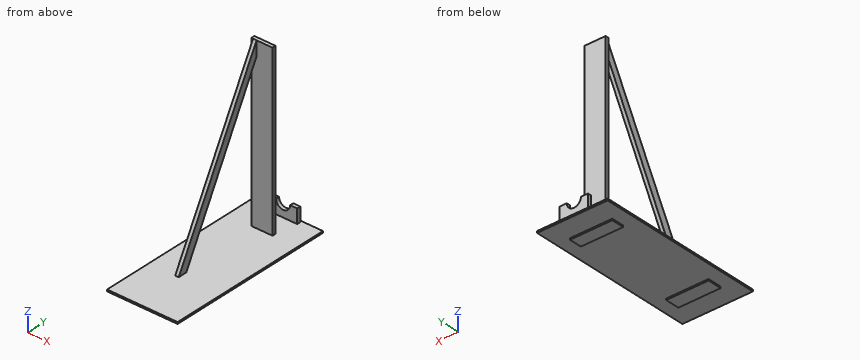
from build123d import *

# Parameters (mm, degrees)
F0_W      = 254
F0_H      = 609.6
F1_DEPTH  = 6.35
F2_W      = 152.4
F2_H      = 50.8
F2_H_2    = 45.6810940742
F3_DEPTH  = 5.08
F5_DEPTH  = 50.8
F6_W      = 76.2
F6_H      = 12.7
F7_DEPTH  = 609.6
F9_DEPTH  = 6.35
F11_DEPTH = 25.4


with BuildPart() as f1:
    # F0 (on Top) → F1 (new body)
    with BuildSketch(Plane.XY):
        with Locations((25.4, 0)):
            Rectangle(F0_W, F0_H)
    extrude(amount=F1_DEPTH)

    # F2 (on face) → F3 (join)
    with BuildSketch(Plane(origin=(0, 0, 0), x_dir=(1, 0, 0), z_dir=(0, 0, -1))):
        with Locations((25.4, 203.2)):
            Rectangle(F2_W, F2_H)
        with Locations((25.4, -203.2)):
            Rectangle(F2_W, F2_H_2)
    extrude(amount=F3_DEPTH)

    # F4 (on face) → F5 (join)
    with BuildSketch(Plane.XY.offset(6.35)):
        Polygon((76.2, 285.75), (76.2, 298.45), (25.4, 298.45), (-25.4, 298.45), (-25.4, 285.75), align=None)
    extrude(amount=F5_DEPTH)

    # F6 (on face) → F7 (join)
    with BuildSketch(Plane.XY.offset(6.35)):
        with Locations((25.4, 203.2)):
            Rectangle(F6_W, F6_H)
    extrude(amount=F7_DEPTH)

    # F8 (on Right) → F9 (join, symmetric)
    with BuildSketch(Plane.YZ):
        Polygon((-133.4145218134, 0), (-101.6, 0), (196.6719031334, 564.3243789673), (196.6719031334, 616.1219477654), align=None)
    extrude(amount=F9_DEPTH, both=True)

    # F10 (on face) → F11 (cut)
    with BuildSketch(Plane(origin=(0, 298.45, 0), x_dir=(-1, 0, 0), z_dir=(0, 1, 0))):
        with BuildLine():
            ThreePointArc((-50.8, 57.15), (-25.4, 31.75), (0, 57.15))
            Line((0, 57.15), (-50.8, 57.15))
        make_face()
    extrude(amount=-F11_DEPTH, mode=Mode.SUBTRACT)


solid = f1.part
Can you work these out from the model? Positions are in its coordinate system, mm. Give positions to 0.01 mm unless a question says otherwise; leave off trailing zeros. Loops run counter-clockwise (first coordinate to the right, second up) from the corner with the lowest first, then second, coordinate; pieces in that order, holes last. Notation, with made-up numbers: (37.5, -19.5) - (61.5, -19.5) arc R11 ccw to (61.5, -3.5) - close; hole circle Ø10 at (-13.5, -40). An arc over 180 degrees is marked (long way). One line per item, written item: value.
(1) If we section it at B-B, the plane y = 98.5: List the corners of the cut face in (x, z) for me.
Verdict:
outline: (-101.6, 0) - (152.4, 0) - (152.4, 6.35) - (-101.6, 6.35) - close; (-6.35, 378.59) - (6.35, 378.59) - (6.35, 432.88) - (-6.35, 432.88) - close
(2) If we section it at A-A, the plane z = 388: List the corners of the cut face in (x, y) for me, plus the area to 3 significant figures.
Verdict:
outline: (-12.7, 196.85) - (63.5, 196.85) - (63.5, 209.55) - (-12.7, 209.55) - close; (-6.35, 74.46) - (6.35, 74.46) - (6.35, 103.48) - (-6.35, 103.48) - close
area: 1,340 mm^2
(3) I need wall thicknesses on line 1 along Z through (x, y) = (38, -12); line 2 along Y through (x, z) = (38.5, 310); line 3 along Z through (x, y) = (20, 203.5). Which ranges of each line are inside material? Lowest first, please.
Verdict:
line 1: 0 to 6.35
line 2: 196.85 to 209.55
line 3: -5.08 to 615.95
(4) If we section it at D-D, the plane x = 84: List the corners of the cut face in (y, z) for me, plus the area to 3 significant figures.
Verdict:
outline: (-304.8, 0) - (-228.6, 0) - (-228.6, -5.08) - (-177.8, -5.08) - (-177.8, 0) - (180.36, 0) - (180.36, -5.08) - (226.04, -5.08) - (226.04, 0) - (304.8, 0) - (304.8, 6.35) - (-304.8, 6.35) - close
area: 4,360 mm^2
(5) I'm going to push flat-ended pins straight in: pin 1 (8 mm diameter, centred on x = 59.5, y = 121, fed in from -Z); pin 2 (10 mm diameter, centred on x = 67, y = -21.5, fed in from +Z); pin 3 (4 mm diameter, centred on x = -7.5, y = 289.5, fed in from +Z). Where does each tip first touch, or does it pass through?
Verdict:
pin 1: z = 0
pin 2: z = 6.35
pin 3: z = 57.15
(6) If we section it at C-C, the plane x = 25.4: List the corners of the cut face in (y, z) for me.
Verdict:
outline: (-304.8, 0) - (-228.6, 0) - (-228.6, -5.08) - (-177.8, -5.08) - (-177.8, 0) - (180.36, 0) - (180.36, -5.08) - (226.04, -5.08) - (226.04, 0) - (304.8, 0) - (304.8, 6.35) - (298.45, 6.35) - (298.45, 31.75) - (285.75, 31.75) - (285.75, 6.35) - (209.55, 6.35) - (209.55, 615.95) - (196.85, 615.95) - (196.85, 6.35) - (-304.8, 6.35) - close
